```python
from build123d import *

# Parameters (mm, degrees)
SKETCH1_R           = 13
BOSS_EXTRUDE1_DEPTH = 3
SKETCH2_R           = 10
BOSS_EXTRUDE2_DEPTH = 4
CHAMFER1_SIZE       = 0.5
SKETCH3_R           = 6
CUT_EXTRUDE1_DEPTH  = 20.672315573


with BuildPart() as part:
    # Sketch1 → Boss-Extrude1 (new body)
    with BuildSketch(Plane(origin=(0, 0, 0), x_dir=(1, 0, 0), z_dir=(0, 1, 0))):
        with Locations(Location((0, 0, 0), (0, 0, 270))):
            Circle(SKETCH1_R)
    extrude(amount=BOSS_EXTRUDE1_DEPTH)

    # Sketch2 → Boss-Extrude2 (add)
    with BuildSketch(Plane.XZ):
        with Locations(Location((0, 0, 0), (0, 0, 270))):
            Circle(SKETCH2_R)
    extrude(amount=BOSS_EXTRUDE2_DEPTH)

    # Chamfer1
    chamfer1_edges = [part.edges().sort_by_distance(p)[0] for p in [
        (0, 0, 10),
        (0, -4, 10),
    ]]
    chamfer(chamfer1_edges, length=CHAMFER1_SIZE)

    # Sketch3 → Cut-Extrude1 (cut, through all)
    with BuildSketch(Plane(origin=(0, 3, 0), x_dir=(1, 0, 0), z_dir=(0, 1, 0))):
        with Locations(Location((0, 0, 0), (0, 0, 270))):
            Circle(SKETCH3_R)
    extrude(amount=-CUT_EXTRUDE1_DEPTH, mode=Mode.SUBTRACT)


solid = part.part
```
Verification items for the finished model (mm, model axes). A direction names the side the tool comes from. Coordinates: 2 decimals unless noted, no trailing zeros. Order: outer loops, then holes, each group sorted by start corner. A loop starts at its lowest first (then second) coordinate and runs counter-clockwise, first axis right, second up. Notation, with made-up numbers: (84, 80.25) -> (130, 80.25) arc R11 cw to (130, 94.25) -> close; hole circle Ø2 at (-32, 78.25). An arc over 180 degrees is marked (long way). Answer as CSV lines item,"result". Start each with the question number.
1) Cross-section at C-C, the plane y = -2. Record the boundary of the cut face in (x, z), then the cut area to 3 significant figures.
2) Gauge pin test, flat ends, axial feed: pin 1 Ø4 at (x, z) = (-4.5, 0) entering from -Y; pin 2 Ø3 at (y, z) = (-3, -2) entering from +X; pin 3 Ø4 at (y, z) = (-3, 10) entering from -X; pin 4 Ø2 at (x, y) = (4, -3) entering from +Z. Record the tip position at first contact, or that the pin passes through.
3) Cross-section at D-D, the plane x = -11. Record the boundary of the cut face in (y, z).
4) Material ranges on L1, parallel to X at y = -2, z = 0; L2, parallel to X at y = 1.75, z = 0; L3, parallel to Y at x = -8.75, z = 8.5, recorded low to high. Write a range as [from, to].
5) Cross-section at B-B, the plane x = 0. Record the boundary of the cut face in (y, z).
6) Set-up check for faces 1 (the face through (-3, 3, 6)), 2 (the face through (-9.76, -1.98, 2.17)): record each of +Z, -Z, +X, -X, +Y, -Y from which the full face is reachable in a straight line by a thin tool's end or side.
7) Cross-section at A-A, the plane z = 0. Record the boundary of the cut face in (x, y).
Conclusion:
1,outline,"circle Ø20 at (0, 0); hole circle Ø12 at (0, 0)"
1,area,"201 mm²"
2,pin 1,"stops at y = -4"
2,pin 2,"stops at x = 9.99"
2,pin 3,"stops at x = -6"
2,pin 4,"stops at z = 9.54"
3,outline,"(0, -6.93) -> (3, -6.93) -> (3, 6.93) -> (0, 6.93) -> close"
4,L1,"x = [-10, -6], [6, 10]"
4,L2,"x = [-13, -6], [6, 13]"
4,L3,"y = [0, 3]"
5,outline,"(-4, -9.5) -> (-3.5, -10) -> (-0.5, -10) -> (0, -10.5) -> (0, -13) -> (3, -13) -> (3, -6) -> (-4, -6) -> close; (-4, 6) -> (3, 6) -> (3, 13) -> (0, 13) -> (0, 10.5) -> (-0.5, 10) -> (-3.5, 10) -> (-4, 9.5) -> close"
6,face 1,"+Z, -Z, +X, -X, +Y"
6,face 2,"-Y"
7,outline,"(-13, 0) -> (-10.5, 0) -> (-10, -0.5) -> (-10, -3.5) -> (-9.5, -4) -> (-6, -4) -> (-6, 3) -> (-13, 3) -> close; (6, -4) -> (9.5, -4) -> (10, -3.5) -> (10, -0.5) -> (10.5, 0) -> (13, 0) -> (13, 3) -> (6, 3) -> close"
